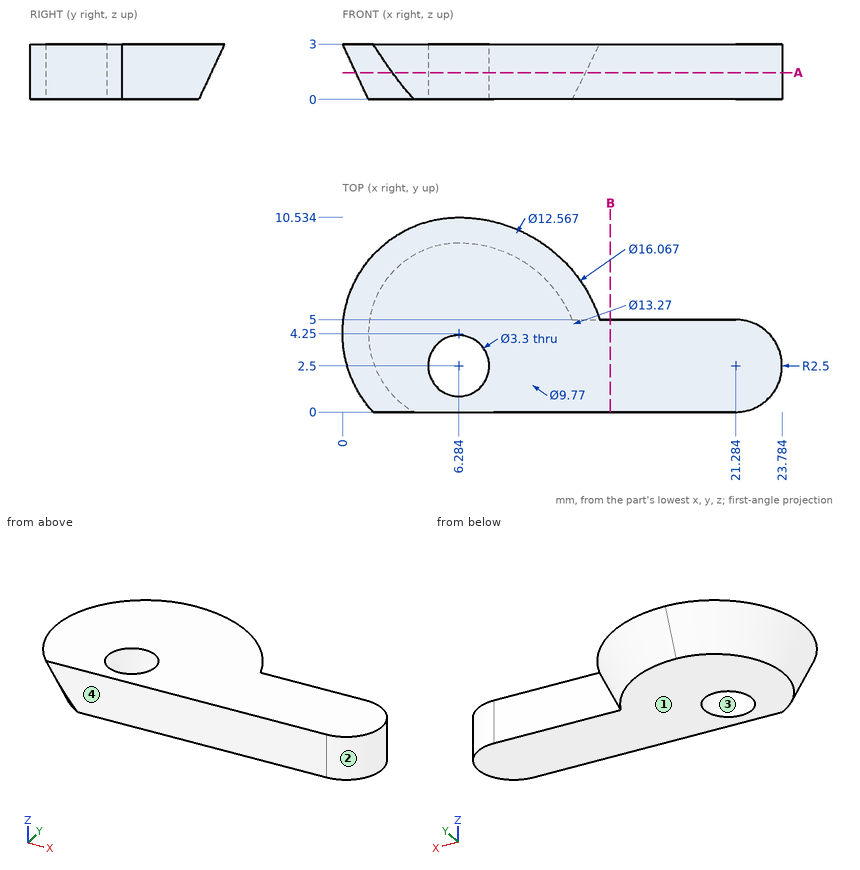
Design review of the part shown in the three views and the two pictorial views. Dimensions are in mm from the part's minimum x, y and z. Round coordinates to 2 decimals unless told otherwise and drop trailing zeros. Loops run counter-clockwise (first coordinate to the right, second up) from the corner with the lowest first, then second, coordinate; pieces in that order, holes last. Notation, with made-up numbers: M 71,5.5 L 96,5.5 A25 cw 96,27.5 Z; hole C 87.25,74.5 d10. An arc over 180 degrees is marked long. Answer as a JSON object with one key per item and string values.
Item 1: We need section B-B, the plane x = 14.5. State the section outline as (y, z) points.
Check sheet entries:
{"outline": "M 0,0 L 5,0 L 5,3 L 0,3 Z"}
Item 2: For line 1 along X through (y, z) = (2, 0.9) (1 decimal); line 2 along Y through (x, z) = (16, 0.9); line 3 along X through (y, z) = (1.75, 2.25) (1 decimal), list the stretches that pass through material, from the lowest coordinate up.
Check sheet entries:
{"line 1": "1.5 to 4.7, 7.9 to 23.7", "line 2": "0 to 5", "line 3": "0.9 to 4.8, 7.8 to 23.7"}
Item 3: The part is to be moulded in two halves that separate along Y. For the marked faces 1, 2, 3 and 4, say which applies: +Y half, -Y half, draft (parallel to the pull), parting line (faces both ways), or undercut.
Check sheet entries:
{"face 1": "draft", "face 2": "parting line", "face 3": "undercut", "face 4": "-Y half"}
Item 4: We need section A-A, the plane z = 1.45. State the section outline as (x, y) points, and give its area (3 significant figures).
Check sheet entries:
{"outline": "M 2.7,0 L 21.28,0 A2.5 ccw 21.28,5 L 13.15,5 A7.31 ccw 6.28,9.81 A5.56 ccw Z; hole C 6.28,2.5 d3.3", "area": "146 mm2"}
Item 5: Clearance check with flat-ended pins moving along their axes: P1, Ø1.5, axis at y = 2.5, z = 2.5, coming from the -X side; P2, Ø2.5, axis at x = 6.28, y = 2.5, coming from the +Z side; P3, Ø1.5, axis at x = 8, y = 9.5, coming from the -Z side. State where each tip first meets the part, or that it passes through.
Check sheet entries:
{"P1": "x = 0.11", "P2": "through", "P3": "z = 0"}
